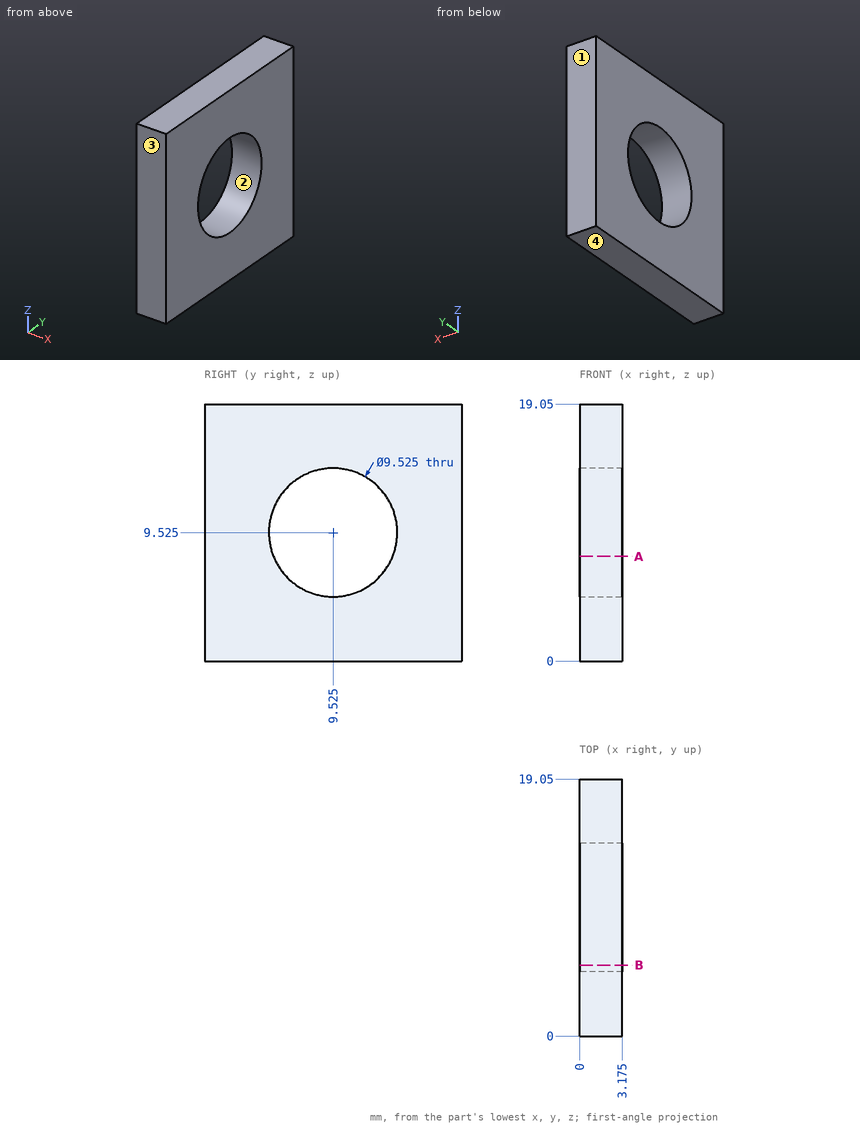
The drawing under review shows one solid part. Ordinate dimensions are in mm from its lowest x, y, z. Round coordinates to 2 decimals unless told otherwise and drop trailing zeros. Write each loop counter-clockwise with the first axis right and the second up, starting at its lowest first coordinate (ties: lowest second). Pieces come first, ordered by that corner, then holes. Notation, with made-up numbers: (0, 73.25) - (22, 73.25) arc R28 cw to (22, 95.25) - close; hole circle Ø10 at (-39, 67.5). An arc over 180 degrees is marked (long way). Use one line per item in the form item = value.
Q1. For line 1 (Z direction, x = 0.3, y = 7.25); line 2 (Z direction, x = 2.15, y = 7.5); line 3 (Y direction, x = 2.65, z = 13.5), list the stretches that pass through material, from the lowest coordinate up. Write a range as [from, to].
Answer key:
line_1 = [0, 5.34], [13.71, 19.05]
line_2 = [0, 5.21], [13.84, 19.05]
line_3 = [0, 6.9], [12.15, 19.05]
Q2. Consider section B-B (y = 5.25). State the section outline as (x, z) points (3 decimals), and give its area (3 significant figures).
Answer key:
outline = (0, 0) - (3.175, 0) - (3.175, 7.426) - (0, 7.426) - close; (0, 11.624) - (3.175, 11.624) - (3.175, 19.05) - (0, 19.05) - close
area = 47.2 mm2
Q3. Draft analysis for pull direction Y (two halves, no side actions). For the marked faces 1, 2, 3 and 4, state which applies: +Y half, -Y half, draft (parallel to the pull), parting line (faces both ways), or undercut.
Answer key:
face_1 = +Y half
face_2 = undercut
face_3 = -Y half
face_4 = draft
Q4. Consider section A-A (z = 7.75). State the section outline as (x, y) points (3 decimals).
Answer key:
outline = (0, 0) - (3.175, 0) - (3.175, 5.106) - (0, 5.106) - close; (0, 13.944) - (3.175, 13.944) - (3.175, 19.05) - (0, 19.05) - close
